from build123d import *

# Parameters (mm, degrees)
SKIZZE1_W                       = 1500
SKIZZE1_H                       = 1000
AUFSATZ_LINEAR_AUSTRAGEN1_DEPTH = 50
SCHNITT_LINEAR_AUSTRAGEN1_REACH = 52
SKIZZE2_W                       = 50
SKIZZE2_H                       = 200
SCHNITT_LINEAR_AUSTRAGEN2_REACH = 52
SKIZZE3_W                       = 50
SKIZZE3_H                       = 200


with BuildPart() as part:
    # Skizze1 → Aufsatz-Linear austragen1 (new body)
    with BuildSketch(Plane.XY):
        with Locations((0, -500)):
            Rectangle(SKIZZE1_W, SKIZZE1_H)
    extrude(amount=AUFSATZ_LINEAR_AUSTRAGEN1_DEPTH)

    # Skizze2 → Schnitt-Linear austragen1 (cut, up to next)
    with BuildSketch(Plane.XY.offset(50), mode=Mode.PRIVATE) as schnitt_linear_austragen1_sk1:
        with Locations((-725, -500)):
            Rectangle(SKIZZE2_W, SKIZZE2_H)
    schnitt_linear_austragen1_tool1 = extrude(schnitt_linear_austragen1_sk1.sketch, amount=-SCHNITT_LINEAR_AUSTRAGEN1_REACH, mode=Mode.PRIVATE) & part.part
    add(schnitt_linear_austragen1_tool1.solids().sort_by_distance((-725, -500, 50))[0], mode=Mode.SUBTRACT)

    # Skizze3 → Schnitt-Linear austragen2 (cut, up to next)
    with BuildSketch(Plane.XY.offset(50), mode=Mode.PRIVATE) as schnitt_linear_austragen2_sk1:
        with Locations((725, -500)):
            Rectangle(SKIZZE3_W, SKIZZE3_H)
    schnitt_linear_austragen2_tool1 = extrude(schnitt_linear_austragen2_sk1.sketch, amount=-SCHNITT_LINEAR_AUSTRAGEN2_REACH, mode=Mode.PRIVATE) & part.part
    add(schnitt_linear_austragen2_tool1.solids().sort_by_distance((725, -500, 50))[0], mode=Mode.SUBTRACT)


solid = part.part
Could you check a few things on this model? Use its own coordinates, in mm. A direction names the side the tool comes from. Round coordinates to 2 decimals unless told otherwise and drop trailing zeros. Order: outer loops, then holes, each group sorted by start corner. A loop starts at its lowest first (then second) coordinate and runs counter-clockwise, first axis right, second up.
(1) Imagine slicing it at A-A (y = -422). Write out the boundary of the cut face in (x, z).
Response values:
outline: (-700, 0) - (700, 0) - (700, 50) - (-700, 50) - close
(2) Please list where this line runs through material, in increasing order: line 1 along X through (y, z) = (-483.5, 38.5).
Response values:
line 1: x = -700 to 700
(3) Which directions (+Z, -Z, +X, -X, +Y, -Y) give clear straight access to the entire face, cutting with the end or side of a thin tool? Please do faces 5 (the flat face through (725, -400, 25)), 6 (the flat face through (-750, -203, 25)), 7 (the flat face through (-725, -400, 25)).
Response values:
face 5: +Z, -Z, +X
face 6: +Z, -Z, -X, +Y, -Y
face 7: +Z, -Z, -X
(4) If we mould it in two halves opening along Y, with no side actions, what happens to faces 1 (the flat face through (-10, -493, 0)), 2 (the flat face through (725, -600, 25)), 3 (the flat face through (-700, -501, 25)), 4 (the flat face through (-10, 0, 25))? For each: released by +Y, released by -Y, zero draft, split by the parting line, or undercut.
Response values:
face 1: zero draft
face 2: undercut
face 3: undercut
face 4: released by +Y
(5) I'm going to push a flat-ended pin straight in: pin 1 (2 mm diameter, centred on y = -461, z = 20.5, fed in from -X). Where does the tip first touch, or does it pass through?
Response values:
pin 1: stops at x = -700
